For this review, use the dimensioned drawing (mm, ordinates from the lowest corner) and the shaded views. A direction names the side the tool comes from. Coordinates: 2 decimals unless noted, no trailing zeros. Write each loop counter-clockwise with the first axis right and the second up, starting at its lowest first coordinate (ties: lowest second). Pieces come first, ordered by that corner, then holes. Notation, with made-up numbers: M -25,30 L -21,30 A33 cw -21,64 Z; hole C 20.5,48 d2. An arc over 180 degrees is marked long. Return JSON: item names as keys, results as strings.
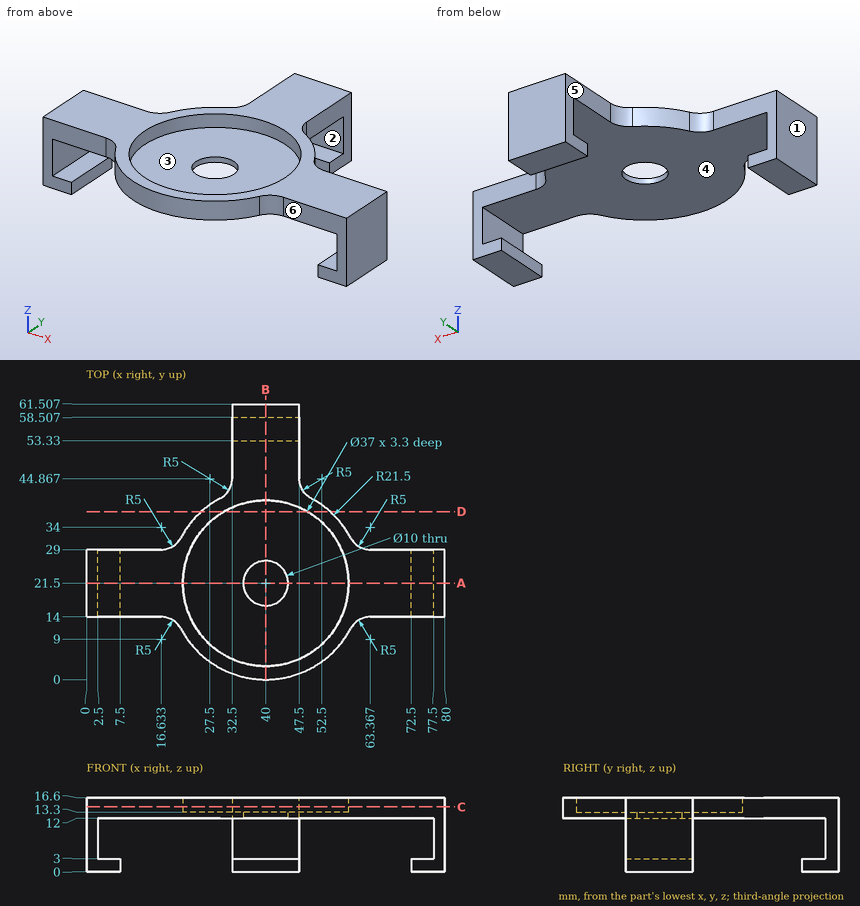
1. We need section A-A (y = 21.5). State the section outline as (x, z) points, plus the area to 3 significant figures.
Checks:
{"outline": "M 0,0 L 7.5,0 L 7.5,3 L 2.5,3 L 2.5,12 L 35,12 L 35,13.3 L 21.5,13.3 L 21.5,16.6 L 0,16.6 Z; M 45,12 L 77.5,12 L 77.5,3 L 72.5,3 L 72.5,0 L 80,0 L 80,16.6 L 58.5,16.6 L 58.5,13.3 L 45,13.3 Z", "area": "323 mm2"}
2. We need section B-B (x = 40). State the section outline as (y, z) points.
Checks:
{"outline": "M 0,12 L 16.5,12 L 16.5,13.3 L 3,13.3 L 3,16.6 L 0,16.6 Z; M 26.5,12 L 58.51,12 L 58.51,3 L 53.33,3 L 53.33,0 L 61.51,0 L 61.51,16.6 L 40,16.6 L 40,13.3 L 26.5,13.3 Z"}
3. We need section C-C (z = 14.5). State the section outline as (x, y) points.
Checks:
{"outline": "M 0,14 L 16.63,14 A5 cw 21.04,11.36 A21.5 ccw 58.96,11.36 A5 cw 63.37,14 L 80,14 L 80,29 L 63.37,29 A5 cw 58.96,31.64 A21.5 ccw 50.14,40.46 A5 cw 47.5,44.87 L 47.5,61.51 L 32.5,61.51 L 32.5,44.87 A5 cw 29.86,40.46 A21.5 ccw 21.04,31.64 A5 cw 16.63,29 L 0,29 Z; hole C 40,21.5 d37"}
4. Wall thickness on L1, parallel to X at y = 21.5, z = 15.3; L2, parallel to Z at x = 73, y = 21.5; L3, parallel to Y at x = 11.5, z = 16: over which ranges is each line inside the solid? List them lowest first. Write a range as from..to.
Checks:
{"L1": "0..21.5, 58.5..80", "L2": "0..3, 12..16.6", "L3": "14..29"}
5. Draft analysis for pull direction Z (two halves, no side actions). For the marked faces 1, 2 and 3, state which applies: +Z half, -Z half, draft (parallel to the pull), parting line (faces both ways), or undercut.
Checks:
{"face 1": "draft", "face 2": "undercut", "face 3": "+Z half"}
6. For the marked faces 4, 5 and 6, list the 3-axis set-ups (+Z, -Z, +X, -X, +Y, -Y) from which the entire face can be reached by the end or side of a thin tool; tool diameter is ignored.
Checks:
{"face 4": "-Y", "face 5": "+Z, -Z, -X, +Y", "face 6": "+Z, -Z, +X, -Y"}
7. We need section D-D (y = 37.5). State the section outline as (x, z) points.
Checks:
{"outline": "M 25.64,12 L 54.36,12 L 54.36,16.6 L 49.29,16.6 L 49.29,13.3 L 30.71,13.3 L 30.71,16.6 L 25.64,16.6 Z"}
8. Clearance check with flat-ended pins moving along their axes: pin 1 Ø5 at (x, z) = (70.5, 12.5) entering from -Y; pin 2 Ø16 at (x, y) = (40, 21.5) entering from -Z; pin 3 Ø8.5 at (y, z) = (55, 5.5) entering from -X. State where each tip first meets the part, or that it passes through.
Checks:
{"pin 1": "y = 14", "pin 2": "z = 12", "pin 3": "x = 32.5"}
